Geometry: see drawing. Coordinates: mm, zero at the bounding-box minimum. A direction names the side the tool comes from. Give positions to 0.01 mm unless a question says otherwise; leave off trailing zeros. Put each result on its own line as item: value.
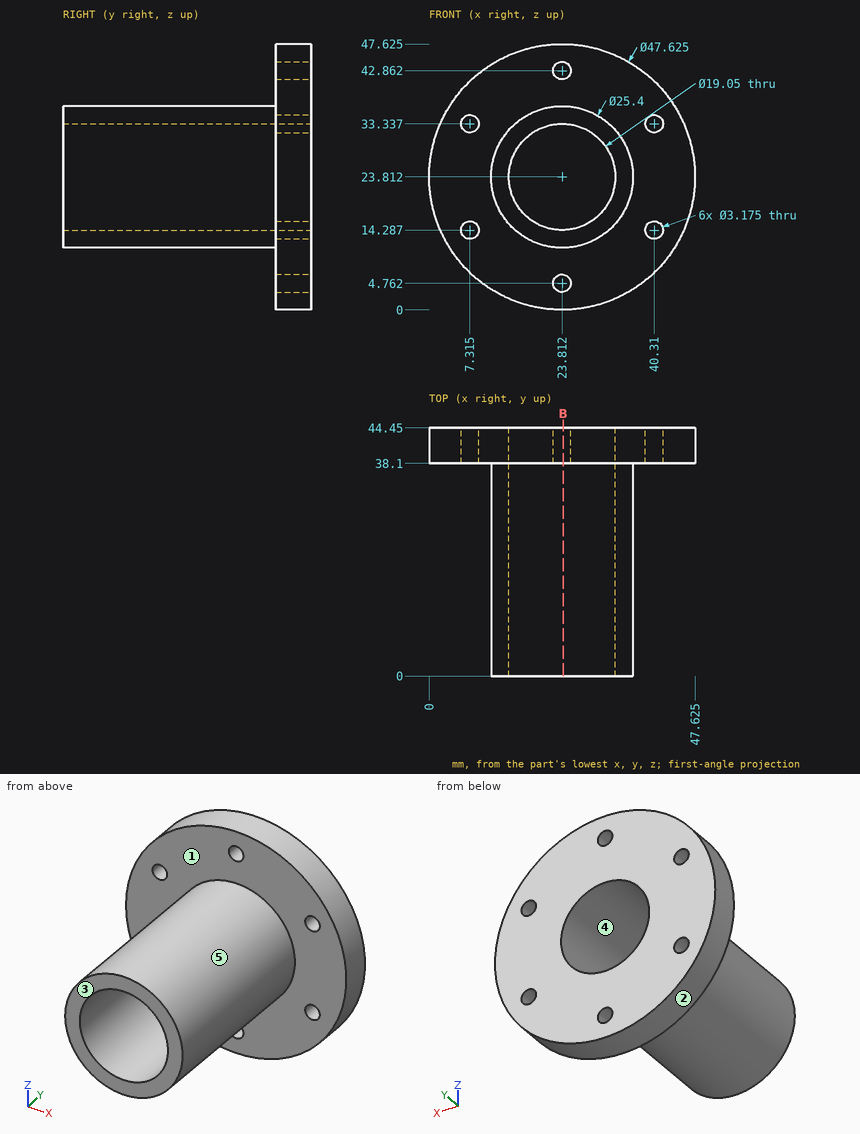
1. Draft query along Z for the marked faces 3, 4 and 5. Return one class per face: pulls with the +Z half, pulls with the -Z half, needs draft (parallel to the pull), parting line crosses it, or undercut.
Found:
face 3: needs draft
face 4: undercut
face 5: parting line crosses it
2. Material intervals for line 1 (X direction, y = 26, z = 24) (1 decimal); line 2 (X direction, y = 23, z = 30) (1 decimal); line 3 (Y direction, x = 11.5, z = 15), sorted ascending. Write a range as from..to.
Found:
line 1: 11.1..14.3, 33.3..36.5
line 2: 12.7..16.6, 31.1..34.9
line 3: 38.1..44.45
3. Section query B-B (x = 24). State how many separate pieces and enclosed holes the cut face has.
Found:
separate pieces: 4
enclosed holes: 0
4. Contact query for flat-ended pins moving along their axis: P1, Ø2.5, axis at x = 7.31, z = 33.34, coming from the +Y side; P2, Ø1, axis at x = 35.5, z = 7, coming from the -Y side; P3, Ø12, axis at x = 8.5, y = 25.5, coming from the -Z side; P4, Ø1.5, axis at y = 24.5, z = 22.5, coming from the -X side (1 decimal). Output: stop coordinate, or through.
Found:
P1: through
P2: y = 38.1
P3: z = 15.18
P4: x = 11.1
5. Access query for the marked faces 1 and 2. Directions: +Z, -Z, +X, -X, +Y, -Y. A direction counts if a zero-diameter tool reaches every point of the face in a straight line with its end or side. Return the directions, or none.
Found:
face 1: -Y
face 2: +Y, -Y
